Input: part model. Units: mm. Frame: model coordinates. Coordinates: 2 decimals unless noted, no trailing zeros. Write each loop counter-clockwise with the first axis right and the second up, starting at its lowest first coordinate (ties: lowest second). Pieces come first, ordered by that corner, then holes. Notation, with made-up numbers: (-13.5, 13) - (-1.5, 13) arc R24 ccw to (-1.5, 51) - close; hole circle Ø6 at (14.5, 67). An arc over 180 degrees is marked (long way). Use a Markdown table: item, result. Add a question column.
Q1. Section query B-B (z = -21.5). Return the cut outline in (x, y), then the cut area to 3 significant figures.
Q2. Material intervals for probe 1 along Z at (x, y) = (0, -11.5); probe 2 along Z at (x, y) = (15.5, -8); probe 3 along X at (y, z) = (-24, -27.5), sorted ascending. Write a range as from..to.
Q3. Section query A-A (x = 0). Return the cut outline in (y, z).
Q4. Pin query (flat end, axial travel): P1, Ø1, axis at y = -22.5, z = 11, coming from the -X side; P2, Ø1.5, axis at y = -36, z = 1.5, coming from the -X side; P3, Ø6, axis at x = -1.5, z = -6.5, coming from the -Y side; P4, Ø1, axis at y = -40, z = 1.5, coming from the -X side. Return the tip coordinate at first contact, or that it passes through.
Q5. Mould query, pull axis X, two halves, no side actions, for faces 1 (the face through (-38.529, -25.756, -53.247)), 2 (the face through (41.65, -25.76, -53.7)), 3 (the face through (1, -25, -64.844)), 4 (the face through (10.17, -25.76, -3.7)). Classes: released by +X, released by -X, zero draft, split by the parting line, or undercut.
Q6. Section query C-C (y = -9.5). Return the cut outline in (x, z).
from build123d import *

# Parameters (mm, degrees)
F0_W     = 103.9975248277
F0_H     = 89.1407411546
F1_DEPTH = 50.8
F2_R     = 18.9210521973
F3_DEPTH = 50.801
F5_DEPTH = 50.801


with BuildPart() as f1:
    # F0 (on Front) → F1 (new body)
    with BuildSketch(Plane.XZ):
        with Locations((1.8570963293, -20.2733287588)):
            Rectangle(F0_W, F0_H)
    extrude(amount=F1_DEPTH)

    # F2 (on face) → F3 (cut, through all)
    with BuildSketch(Plane.XZ.offset(50.8)):
        with Locations((0, -19.6542944759)):
            Circle(F2_R)
    extrude(amount=-F3_DEPTH, mode=Mode.SUBTRACT)

    # F4 (on face) → F5 (cut, through all)
    with BuildSketch(Plane.XZ.offset(50.8)):
        Polygon((-50.1416660845, 24.2970418185), (-50.1416660845, 0), (-29.0945451707, 24.2970418185), align=None)
        Polygon((53.8558587432, 24.2970418185), (33.7372943759, 24.2970418185), (53.8558587432, 0), align=None)
        Polygon((-27.2374469787, -64.8436993361), (-50.1416660845, -41.3204431534), (-50.1416660845, -64.8436993361), align=None)
        Polygon((53.8558587432, -42.8680256009), (29.094548896, -64.8436993361), (53.8558587432, -64.8436993361), align=None)
    extrude(amount=-F5_DEPTH, mode=Mode.SUBTRACT)


solid = f1.part
Values follow:
| question | item | result |
|---|---|---|
| 1 | outline | (-50.14, -50.8) - (-18.83, -50.8) - (-18.83, 0) - (-50.14, 0) - close; (18.83, -50.8) - (53.86, -50.8) - (53.86, 0) - (18.83, 0) - close |
| 1 | area | 3,370 mm2 |
| 2 | probe 1 | -64.84..-38.58, -0.73..24.3 |
| 2 | probe 2 | -64.84..-30.51, -8.8..24.3 |
| 2 | probe 3 | -50.14..-17.22, 17.22..53.86 |
| 3 | outline | (-50.8, -64.84) - (0, -64.84) - (0, -38.58) - (-50.8, -38.58) - close; (-50.8, -0.73) - (0, -0.73) - (0, 24.3) - (-50.8, 24.3) - close |
| 4 | P1 | x = -41.05 |
| 4 | P2 | x = -49.49 |
| 4 | P3 | through |
| 4 | P4 | x = -49.28 |
| 5 | face 1 | released by -X |
| 5 | face 2 | released by +X |
| 5 | face 3 | zero draft |
| 5 | face 4 | undercut |
| 6 | outline | (-50.14, -41.32) - (-27.24, -64.84) - (29.09, -64.84) - (53.86, -42.87) - (53.86, 0) - (33.74, 24.3) - (-29.09, 24.3) - (-50.14, 0) - close; hole circle Ø37.84 at (0, -19.65) |
